Geometry check sheet. Reference: the model listing, model coordinates, mm. A direction names the side the tool comes from. Coordinates: 2 decimals unless noted, no trailing zeros. Write each loop counter-clockwise with the first axis right and the second up, starting at its lowest first coordinate (ties: lowest second). Pieces come first, ordered by that corner, then holes. Notation, with made-up numbers: M 59.25,41.25 L 66.25,41.25 A23 ccw 66.25,50.25 Z; hole C -17.75,-29.75 d5. An arc over 180 degrees is marked long. Write each question's results on one line, items separated by ' | '.
```python
from build123d import *

# Parameters (mm, degrees)
F0_W     = 19.2
F0_H     = 19.2
F1_DEPTH = 19.2
F2_W     = 15.3
F2_H     = 15.3
F3_DEPTH = 16.4
F4_SIZE  = 0.6
F5_R     = 0.6
F6_SIZE  = 0.3


with BuildPart() as f1:
    # F0 (on Top) → F1 (new body)
    with BuildSketch(Plane.XY):
        Rectangle(F0_W, F0_H)
    extrude(amount=F1_DEPTH)

    # F2 (on face) → F3 (cut)
    with BuildSketch(Plane(origin=(0, 0, 0), x_dir=(1, 0, 0), z_dir=(0, 0, -1))):
        Rectangle(F2_W, F2_H)
    extrude(amount=-F3_DEPTH, mode=Mode.SUBTRACT)

    # F4
    f4_edges = [f1.edges().sort_by_distance(p)[0] for p in [
        (-9.6, -9.6, 9.6),
        (-9.6, 9.6, 9.6),
        (9.6, 9.6, 9.6),
        (9.6, -9.6, 9.6),
        (0, -9.6, 19.2),
        (9.6, 0, 19.2),
        (0, 9.6, 19.2),
        (-9.6, 0, 19.2),
    ]]
    chamfer(f4_edges, length=F4_SIZE)

    # F5
    f5_edges = [f1.edges().sort_by_distance(p)[0] for p in [
        (-7.65, 7.65, 8.2),
        (-7.65, -7.65, 8.2),
        (7.65, -7.65, 8.2),
        (7.65, 7.65, 8.2),
        (7.65, 0, 16.4),
        (0, -7.65, 16.4),
        (-7.65, 0, 16.4),
        (0, 7.65, 16.4),
    ]]
    fillet(f5_edges, radius=F5_R)

    # F6
    f6_edges = [f1.edges().sort_by_distance(p)[0] for p in [
        (0, 7.65, 0),
        (-7.474264, 7.474264, 0),
        (7.474264, 7.474264, 0),
        (-7.65, 0, 0),
        (7.65, 0, 0),
        (-7.474264, -7.474264, 0),
        (7.474264, -7.474264, 0),
        (0, -7.65, 0),
        (0, -9.6, 0),
        (-9.3, -9.3, 0),
        (9.3, -9.3, 0),
        (-9.6, 0, 0),
        (9.6, 0, 0),
        (-9.3, 9.3, 0),
        (9.3, 9.3, 0),
        (0, 9.6, 0),
    ]]
    chamfer(f6_edges, length=F6_SIZE)


solid = f1.part
```
Q1. Sectioned sample at A-A on z = 6.75. Record the cut outline in (x, y), and give its area (3 significant figures).
Geometry check:
outline: M -9.6,-9 L -9,-9.6 L 9,-9.6 L 9.6,-9 L 9.6,9 L 9,9.6 L -9,9.6 L -9.6,9 Z; hole M -7.65,-7.05 A0.6 ccw -7.05,-7.65 L 7.05,-7.65 A0.6 ccw 7.65,-7.05 L 7.65,7.05 A0.6 ccw 7.05,7.65 L -7.05,7.65 A0.6 ccw -7.65,7.05 Z | area: 134 mm2
Q2. Scan lines: probe 1 along X at (y, z) = (5, 13); probe 2 along Z at (x, y) = (-4.75, 0.5). Record each from-to range of solid material in increasing order.
Geometry check:
probe 1: x = -9.6 to -7.65, 7.65 to 9.6 | probe 2: z = 16.4 to 19.2
Q3. Mould release check, pull along Y, two halves, no side actions. Record for faces 1 (the flat face through (-9.6, 0, 9)), 2 (the flat face through (7.65, 0, 8)), 3 (the flat face through (0, 9.6, 9)): pulls with the +Y half, pulls with the -Y half, needs draft (parallel to the pull), parting line crosses it, or undercut.
Geometry check:
face 1: needs draft | face 2: undercut | face 3: pulls with the +Y half
Q4. Depth check by flat-ended pin: P1, Ø4, axis at x = 0, y = -2.5, coming from the -Z side. Enter the tip coordinate at first touch or a pass-through.
Geometry check:
P1: stops at z = 16.4
Q5. Access from +Z, -Z, +X, -X, +Y, -Y to the whole of each face (thin tool, end or side, straight path). Record for faces 4 (the flat face through (9.6, 0, 9)), 5 (the flat face through (0, 7.65, 8)).
Geometry check:
face 4: +Z, -Z, +X, +Y, -Y | face 5: -Z
Q6. Sectioned sample at B-B on y = -3. Record the cut outline in (x, z).
Geometry check:
outline: M -9.6,0.3 L -9.3,0 L -7.95,0 L -7.65,0.3 L -7.65,15.8 A0.6 cw -7.05,16.4 L 7.05,16.4 A0.6 cw 7.65,15.8 L 7.65,0.3 L 7.95,0 L 9.3,0 L 9.6,0.3 L 9.6,18.6 L 9,19.2 L -9,19.2 L -9.6,18.6 Z
